from build123d import *

# Parameters (mm, degrees)
SKETCH1_W           = 48
SKETCH1_H           = 48
BOSS_EXTRUDE1_DEPTH = 28
SKETCH2_W           = 38
SKETCH2_H           = 38
CUT_EXTRUDE1_DEPTH  = 29
SKETCH3_W           = 41
SKETCH3_H           = 16.4
CUT_EXTRUDE2_DEPTH  = 2.5
SKETCH4_W           = 3.6
SKETCH4_H           = 10.7
CUT_EXTRUDE3_DEPTH  = 38.5
CUT_EXTRUDE4_REACH  = 50
CUT_EXTRUDE5_DEPTH  = 42.2
CUT_EXTRUDE6_DEPTH  = 46.5
FILLET1_R           = 6
FILLET2_R           = 0.5
FILLET3_R           = 1
FILLET4_R           = 2.5


with BuildPart() as part:
    # Sketch1 → Boss-Extrude1 (new body)
    with BuildSketch(Plane(origin=(0, 28, 0), x_dir=(1, 0, 0), z_dir=(0, 1, 0))):
        with Locations((24, -24)):
            Rectangle(SKETCH1_W, SKETCH1_H)
    extrude(amount=-BOSS_EXTRUDE1_DEPTH)

    # Sketch2 → Cut-Extrude1 (cut, through all)
    with BuildSketch(Plane(origin=(0, 28, 0), x_dir=(-1, 0, 0), z_dir=(0, 1, 0))):
        with Locations((-29, 29)):
            Rectangle(SKETCH2_W, SKETCH2_H)
    extrude(amount=-CUT_EXTRUDE1_DEPTH, mode=Mode.SUBTRACT)

    # Sketch3 → Cut-Extrude2 (cut)
    with BuildSketch(Plane(origin=(0, 0, 0), x_dir=(-1, 0, 0), z_dir=(0, 0, -1))):
        with Locations((-20.5, 14)):
            Rectangle(SKETCH3_W, SKETCH3_H)
    extrude(amount=-CUT_EXTRUDE2_DEPTH, mode=Mode.SUBTRACT)

    # Sketch4 → Cut-Extrude3 (cut)
    with BuildSketch(Plane(origin=(0, 0, 2.5), x_dir=(-1, 0, 0), z_dir=(0, 0, -1))):
        with Locations((-5, 14)):
            Rectangle(SKETCH4_W, SKETCH4_H)
    extrude(amount=-CUT_EXTRUDE3_DEPTH, mode=Mode.SUBTRACT)

    # Sketch5 → Cut-Extrude4 (cut, up to next)
    with BuildSketch(Plane.ZY, mode=Mode.PRIVATE) as cut_extrude4_sk1:
        with BuildLine():
            Line((2.5, 17.05), (2.5, 10.95))
            Line((2.5, 10.95), (34, 10.95))
            ThreePointArc((34, 10.95), (37.05, 14), (34, 17.05))
            Line((34, 17.05), (2.5, 17.05))
        make_face()
    cut_extrude4_tool1 = extrude(cut_extrude4_sk1.sketch, amount=-CUT_EXTRUDE4_REACH, mode=Mode.PRIVATE) & part.part
    add(cut_extrude4_tool1.solids().sort_by_distance((0, 14, 19.454568))[0], mode=Mode.SUBTRACT)

    # Sketch6 → Cut-Extrude5 (cut, through all)
    with BuildSketch(Plane.ZY.offset(-6.8)):
        with BuildLine():
            Line((34, 17.05), (24, 17.05))
            ThreePointArc((24, 17.05), (20.95, 14), (24, 10.95))
            Line((24, 10.95), (34, 10.95))
            ThreePointArc((34, 10.95), (37.05, 14), (34, 17.05))
        make_face()
    extrude(amount=-CUT_EXTRUDE5_DEPTH, mode=Mode.SUBTRACT)

    # Sketch7 → Cut-Extrude6 (cut, through all)
    with BuildSketch(Plane(origin=(0, 0, 2.5), x_dir=(-1, 0, 0), z_dir=(0, 0, -1))):
        with BuildLine():
            Line((-17, 18.5), (-34, 18.5))
            ThreePointArc((-34, 18.5), (-38.5, 14), (-34, 9.5))
            Line((-34, 9.5), (-17, 9.5))
            ThreePointArc((-17, 9.5), (-12.5, 14), (-17, 18.5))
        make_face()
    extrude(amount=-CUT_EXTRUDE6_DEPTH, mode=Mode.SUBTRACT)

    # Fillet1
    fillet1_edges = [part.edges().sort_by_distance(p)[0] for p in [
        (48, 28, 5),
        (48, 0, 5),
        (5, 28, 48),
        (5, 0, 48),
    ]]
    fillet(fillet1_edges, radius=FILLET1_R)

    # Fillet2
    fillet2_edges = [part.edges().sort_by_distance(p)[0] for p in [
        (10, 14, 10),
        (6.8, 8.65, 21.75),
        (6.8, 19.35, 21.75),
        (3.2, 8.65, 21.75),
    ]]
    fillet(fillet2_edges, radius=FILLET2_R)

    # Fillet3
    fillet3_edges = [part.edges().sort_by_distance(p)[0] for p in [
        (0, 14, 48),
        (21, 0, 0),
        (0, 26.242640687, 46.242640687),
        (0, 1.757359313, 46.242640687),
        (21, 28, 0),
        (48, 14, 0),
        (46.242640687, 26.242640687, 0),
        (46.242640687, 1.757359313, 0),
        (0, 0, 21),
        (0, 28, 21),
    ]]
    fillet(fillet3_edges, radius=FILLET3_R)

    # Fillet4
    fillet4_edges = [part.edges().sort_by_distance(p)[0] for p in [
        (10, 14, 48),
        (10, 26.242640687, 46.242640687),
        (10, 1.757359313, 46.242640687),
        (26.25, 0, 10),
        (26.25, 28, 10),
        (48, 14, 10),
        (46.242640687, 26.242640687, 10),
        (46.242640687, 1.757359313, 10),
        (10, 0, 26.25),
        (10, 28, 26.25),
        (10.146446609, 28, 10.146446609),
        (10.146446609, 0, 10.146446609),
    ]]
    fillet(fillet4_edges, radius=FILLET4_R)


solid = part.part
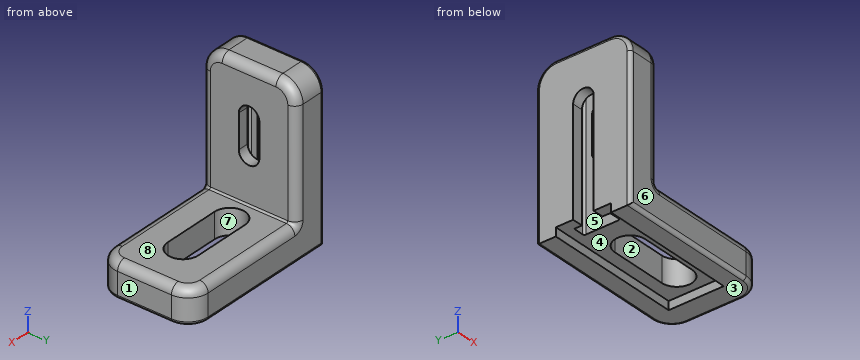
Build history of the part. All positions in model axes, mm. Face numbers are marked on the shaded views. A direction names the side the tool comes from. Round coordinates to 2 decimals unless told otherwise and drop trailing zeros. Write each loop counter-clockwise with the first axis right and the second up, starting at its lowest first coordinate (ties: lowest second). Pieces come first, ordered by that corner, then holes. Notation, with made-up numbers: M 87.25,17.5 L 119.25,17.5 A16 cw 119.25,33.5 Z; hole C 56.5,4 d2. An arc over 180 degrees is marked long. Use CSV: the item, a comma, the result in double quotes.
1. Flat gauge pins, fed straight in: pin 1 (1.5 mm diameter, centred on x = 35, y = 25, fed in from +Z); pin 2 (1 mm diameter, centred on x = 9, z = 30, fed in from +Y); pin 3 (8 mm diameter, centred on y = 13.5, z = 15.5, fed in from +X). Where does each tip first touch, or does it go through?
Reply:
pin 1,"stops at z = 10"
pin 2,"stops at y = 27.79"
pin 3,"stops at x = 10"
2. Saw through at C-C (z = 40). Give the cut face in (x, y), plus the area to 3 significant figures.
Reply:
outline,"M 0,1 A1 ccw 1,0 L 7.5,0 A2.5 ccw 10,2.5 L 10,25.5 A2.5 ccw 7.5,28 L 1,28 A1 ccw 0,27 Z; hole M 3.2,9.15 A0.5 ccw 3.7,8.65 L 6.3,8.65 A0.5 ccw 6.8,9.15 L 6.8,18.85 A0.5 ccw 6.3,19.35 L 3.2,19.35 Z"
area,"239 mm²"
3. Saw through at D-D (y = 21). Give the cut face in (x, z), plus the area to 3 significant figures.
Reply:
outline,"M 0,2.5 L 41,2.5 L 41,0 L 47,0 A1 ccw 48,1 L 48,7.5 A2.5 ccw 45.5,10 L 10.5,10 A0.5 cw 10,10.5 L 10,45.5 A2.5 ccw 7.5,48 L 1,48 A1 ccw 0,47 Z"
area,"754 mm²"
4. Tool access for the marked faces 4, 5, 6, 7 and 8: list every direction of +Z, -Z, +X, -X, +Y, -Y with a clear straight run to the whole face (end or side of a thin tool).
Reply:
face 4,"-Z, -X"
face 5,"-Z"
face 6,"+Z, -Z, +X, -X, -Y"
face 7,"+Z, -Z"
face 8,"+Z, +X, +Y, -Y"
5. Saw through at A-A (x = 18). Give the cut face in (y, z), plus the area to 3 significant figures.
Reply:
outline,"M 0,1 A1 ccw 1,0 L 5.8,0 L 5.8,2.5 L 9.5,2.5 L 9.5,10 L 2.5,10 A2.5 ccw 0,7.5 Z; M 18.5,2.5 L 22.2,2.5 L 22.2,0 L 27,0 A1 ccw 28,1 L 28,7.5 A2.5 ccw 25.5,10 L 18.5,10 Z"
area,"168 mm²"
6. Wall check: probe 1 along X at (y, z) = (16.5, 36); probe 2 along Z at (x, y) = (22.5, 23.75). Give the ranges that are in metal, low to high. Write a range as from..to.
Reply:
probe 1,"x = 0..3.2, 6.8..10"
probe 2,"z = 0..10"
7. Saw through at B-B (y = 14). Give the cut face in (x, z).
Reply:
outline,"M 0,37.05 L 3.2,37.05 L 3.2,41 L 6.8,41 L 6.8,37.05 L 10,37.05 L 10,45.5 A2.5 ccw 7.5,48 L 1,48 A1 ccw 0,47 Z; M 6.8,2.5 L 12.5,2.5 L 12.5,10 L 10.5,10 A0.5 cw 10,10.5 L 10,20.95 L 6.8,20.95 Z; M 38.5,2.5 L 41,2.5 L 41,0 L 47,0 A1 ccw 48,1 L 48,7.5 A2.5 ccw 45.5,10 L 38.5,10 Z"
8. Two-plate mould, pull along X, no slides. Class the marked faces 1, 2 and 3: +X half, -X half, draft (parallel to the pull), parting line (faces both ways), or undercut.
Reply:
face 1,"+X half"
face 2,"undercut"
face 3,"draft"
